```python
from build123d import *

# Parameters (mm, degrees)
F0_R     = 2.5527
F0_R_2   = 1.5875
F1_DEPTH = 2.8448


with BuildPart() as f1:
    # F0 (on Top) → F1 (new body)
    with BuildSketch(Plane.XY):
        with BuildLine():
            Line((27.039664, 30.710469), (-27.720269, 30.710469))
            ThreePointArc((-27.720269, 30.710469), (-28.563817, 31.031086), (-28.981449, 31.831057))
            ThreePointArc((-28.981449, 31.831057), (-45.175495, 37.445661), (-39.560891, 21.251615))
            ThreePointArc((-39.560891, 21.251615), (-38.76092, 20.833983), (-38.440302, 19.990435))
            Line((-38.440302, 19.990435), (-38.440302, -34.769498))
            ThreePointArc((-38.440302, -34.769498), (-38.76092, -35.613046), (-39.560891, -36.030678))
            ThreePointArc((-39.560891, -36.030678), (-45.175495, -52.224723), (-28.981449, -46.61012))
            ThreePointArc((-28.981449, -46.61012), (-28.563817, -45.810149), (-27.720269, -45.489531))
            Line((-27.720269, -45.489531), (27.039664, -45.489531))
            ThreePointArc((27.039664, -45.489531), (27.883212, -45.810149), (28.300844, -46.61012))
            ThreePointArc((28.300844, -46.61012), (44.49489, -52.224723), (38.880286, -36.030678))
            ThreePointArc((38.880286, -36.030678), (38.080315, -35.613046), (37.759698, -34.769498))
            Line((37.759698, -34.769498), (37.759698, 19.990435))
            ThreePointArc((37.759698, 19.990435), (38.080315, 20.833983), (38.880286, 21.251615))
            ThreePointArc((38.880286, 21.251615), (44.49489, 37.445661), (28.300844, 31.831057))
            ThreePointArc((28.300844, 31.831057), (27.883212, 31.031086), (27.039664, 30.710469))
        make_face()
        with Locations((-38.440302, -45.489531)):
            Circle(F0_R, mode=Mode.SUBTRACT)
        with Locations((-21.61768, -20.452246)):
            Circle(F0_R_2, mode=Mode.SUBTRACT)
        with Locations((37.759698, -45.489531)):
            Circle(F0_R, mode=Mode.SUBTRACT)
        with Locations((29.18232, -20.452246)):
            Circle(F0_R_2, mode=Mode.SUBTRACT)
        with BuildLine():
            ThreePointArc((-31.482945, 12.370435), (-29.623073, 16.860563), (-25.132945, 18.720435))
            Line((-25.132945, 18.720435), (19.419664, 18.720435))
            ThreePointArc((19.419664, 18.720435), (23.909792, 16.860563), (25.769664, 12.370435))
            Line((25.769664, 12.370435), (25.769664, -10.966996))
            ThreePointArc((25.769664, -10.966996), (23.909792, -15.457124), (19.419664, -17.316996))
            Line((19.419664, -17.316996), (-25.132945, -17.316996))
            ThreePointArc((-25.132945, -17.316996), (-29.623073, -15.457124), (-31.482945, -10.966996))
            Line((-31.482945, -10.966996), (-31.482945, 12.370435))
        make_face(mode=Mode.SUBTRACT)
        with Locations((-38.440302, 30.710469)):
            Circle(F0_R, mode=Mode.SUBTRACT)
        with Locations((-21.61768, 22.727754)):
            Circle(F0_R_2, mode=Mode.SUBTRACT)
        with Locations((29.18232, 7.487754)):
            Circle(F0_R_2, mode=Mode.SUBTRACT)
        with Locations((37.759698, 30.710469)):
            Circle(F0_R, mode=Mode.SUBTRACT)
    extrude(amount=F1_DEPTH)


solid = f1.part
```
Design review of the part built by this model. Coordinates are the model's own, in mm. A direction names the side the tool comes from. Give positions to 0.01 mm unless a question says otherwise; leave off trailing zeros. Loops run counter-clockwise (first coordinate to the right, second up) from the corner with the lowest first, then second, coordinate; pieces in that order, holes last. Notation, with made-up numbers: M -2.75,88.5 L 51.25,88.5 A21 ccw 51.25,118.5 Z; hole C 32,52 d8. An arc over 180 degrees is marked long. Return JSON: item names as keys, results as strings. Group by question number.
Item 1: For probe 1 along X at (y, z) = (30.5, 2.1); probe 2 along Y at (x, z) = (11, 0.4); probe 3 along X at (y, z) = (-3.5, 1.15), list the stretches that pass through material, from the lowest coordinate up.
Item 2: Insertion check: pin 1 Ø3 at (x, y) = (29.18, -20.45) entering from -Z; pin 2 Ø1 at (x, z) = (-12, 1) entering from +Y; pin 3 Ø1.4 at (y, z) = (-17.5, 1.5) entering from +X. Each pin has a flat end and moves straight along its axis. Give the tip position at first contact, or say it passes through.
Item 3: Mouldability with a two-part tool opening along X and no side actions: class faces 4 (the flat face through (-1, -28, 2.845)), 5 (the flat face through (-38.44, -7, 1)), 6 (the cylindrical face through (38.938, -47.754, 1.402)) as released by +X, released by -X, zero draft, split by the parting line, or undercut.
Item 4: We need section C-C (z = 0.9). Give the number of separate pieces and of enclosed holes in the cut face, and give its area (3 significant figures).
Item 5: We need section D-D (y = -29.5). Give the boundary of the cut face in (x, z), and give its area (3 significant figures).
Item 6: We need section B-B (y = 16). Give the boundary of the cut face in (x, z), and give its area (3 significant figures).
Item 7: We need section A-A (x = 3). Give the boundary of the cut face in (y, z).
Item 8: Tool access review of faces 1 (the flat face through (-1, -45.49, 1)), 2 (the flat face through (25.77, 1, 1)), 3 (the flat face through (0, 30.71, 1)): name each direction out of +Z, -Z, +X, -X, +Y, -Y from which nothing blocks a thin tool from reaching the whole face with its end or side.
Output:
{
 "1": {"probe 1": "x = -47.96 to -40.98, -35.9 to 35.22, 40.3 to 47.28", "probe 2": "y = -45.49 to -17.32, 18.72 to 30.71", "probe 3": "x = -38.44 to -31.48, 25.77 to 37.76"},
 "2": {"pin 1": "passes through", "pin 2": "stops at y = 30.71", "pin 3": "stops at x = 37.76"},
 "3": {"face 4": "zero draft", "face 5": "released by -X", "face 6": "undercut"},
 "4": {"separate pieces": "1", "enclosed holes": "9", "area": "4,520 mm^2"},
 "5": {"outline": "M -38.44,0 L 37.76,0 L 37.76,2.84 L -38.44,2.84 Z", "area": "217 mm^2"},
 "6": {"outline": "M -38.44,0 L -30.34,0 L -30.34,2.84 L -38.44,2.84 Z; M 24.63,0 L 37.76,0 L 37.76,2.84 L 24.63,2.84 Z", "area": "60.4 mm^2"},
 "7": {"outline": "M -45.49,0 L -17.32,0 L -17.32,2.84 L -45.49,2.84 Z; M 18.72,0 L 30.71,0 L 30.71,2.84 L 18.72,2.84 Z"},
 "8": {"face 1": "+Z, -Z, -Y", "face 2": "+Z, -Z", "face 3": "+Z, -Z, +Y"}
}
